```python
from build123d import *

# Parameters (mm, degrees)
F2_SIZE  = 0.762
F4_D     = 5.1054
F4_DEPTH = 25.4
F4_TIP   = 1.5338169022


with BuildPart() as f1:
    # F0 (on Front) → F1 (revolve)
    with BuildSketch(Plane.XZ):
        Polygon((4.7625, 0), (76.2, 0), (76.2, 5.55625), (0, 5.55625), (0, 0), (3.175, 0), (3.175, 3.5687), (4.7625, 3.5687), align=None)
    revolve(axis=Axis((38.1, 0, 5.55625), (1, 0, 0)))

    # F2
    f2_edges = [f1.edges().sort_by_distance(p)[0] for p in [
        (0, 0, 11.1125),
        (76.2, 0, 11.1125),
    ]]
    chamfer(f2_edges, length=F2_SIZE)

    # F4
    with Locations(Plane.YZ.offset(76.2)):
        with Locations((0, 5.55625)):
            Hole(F4_D / 2, depth=F4_DEPTH)
            with Locations((0, 0, -(F4_DEPTH + F4_TIP / 2))):  # 118° drill point
                Cone(0, F4_D / 2, F4_TIP, mode=Mode.SUBTRACT)


solid = f1.part
```
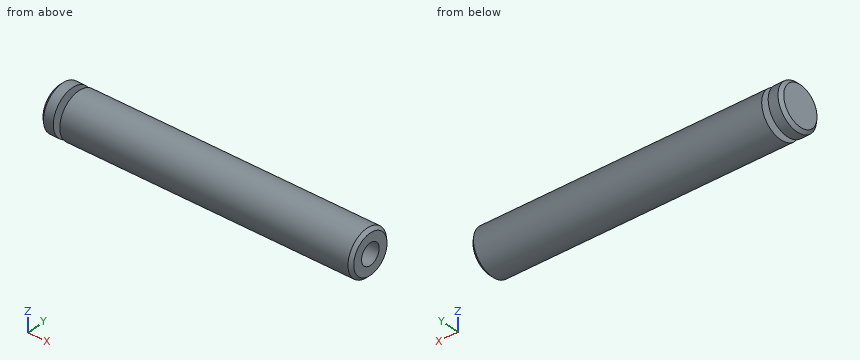
Geometry check sheet. Reference: the model listing, model coordinates, mm. Round coordinates to 2 decimals unless told otherwise and drop trailing zeros. Order: outer loops, then holes, each group sorted by start corner. A loop starts at its lowest first (then second) coordinate and runs counter-clockwise, first axis right, second up. Notation, with made-up numbers: (15.25, 24) - (66.25, 24) arc R7 ccw to (66.25, 36) - close; hole circle Ø3 at (-2, 87). An arc over 180 degrees is marked (long way). Use a Markdown table: item, result. Add a question column.
(1) Sectioned sample at A-A, the plane x = 54. Enter the section's corners in (y, z).
(2) Depth check by flat-ended pin: pin 1 (2 mm diameter, centred on x = 57.5, y = 2.5, fed in from -Z); pin 2 (2 mm diameter, centred on x = 20, z = 4, fed in from +Y). Enter the tip coordinate at first touch or a pass-through.
(3) Material ranges on line 1 along X through (y, z) = (-1, 2.25) (1 decimal); line 2 along X through (y, z) = (-2, 5.25) (1 decimal); line 3 along Y through (x, z) = (53, 3.75), recorded low to high. Write a range as [from, to].
(4) Sectioned sample at B-B, the plane x = 27. Enter the section's corners in (y, z), and give its area (3 significant figures).
Answers below:
| question | item | result |
|---|---|---|
| 1 | outline | circle Ø11.11 at (0, 5.56); hole circle Ø5.11 at (0, 5.56) |
| 2 | pin 1 | z = 0.21 |
| 2 | pin 2 | y = 5.53 |
| 3 | line 1 | [0, 3.2], [4.8, 76.2] |
| 3 | line 2 | [0, 3.2], [4.8, 50.5] |
| 3 | line 3 | [-5.25, -1.8], [1.8, 5.25] |
| 4 | outline | circle Ø11.11 at (0, 5.56) |
| 4 | area | 97.0 mm² |
